from build123d import *

# Parameters (mm, degrees)
ESQUISSE1_R                  = 23
ESQUISSE1_R_2                = 10
BOSS_EXTRU_1_DEPTH           = 8
ENL_V_MAT_EXTRU_1_DEPTH      = 3
ENL_V_MAT_EXTRU_1_DEPTH_BACK = 1
ESQUISSE4_R                  = 4
ENL_V_MAT_EXTRU_2_DEPTH      = 9
R_P_TITION_CIRCULAIRE1_COUNT = 4


with BuildPart() as part:
    # Esquisse1 → Boss.-Extru.1 (new body)
    with BuildSketch(Plane(origin=(0, 0, 0), x_dir=(1, 0, 0), z_dir=(0, 1, 0))):
        with Locations(Location((0, 0, 0), (0, 0, 270))):  # turned: the seam where the file's is
            Circle(ESQUISSE1_R)
        with Locations(Location((0, 0, 0), (0, 0, 270))):  # turned: the seam where the file's is
            Circle(ESQUISSE1_R_2, mode=Mode.SUBTRACT)
    extrude(amount=BOSS_EXTRU_1_DEPTH)

    # Esquisse2 → Enlèv. mat.-Extru.1 (cut, two sides)
    with BuildSketch(Plane.XY.offset(10)) as enl_v_mat_extru_1_sk:
        with BuildLine():
            Line((-3, 0), (-3, 12))
            ThreePointArc((-3, 12), (0, 15), (3, 12))
            Line((3, 12), (3, 0))
            ThreePointArc((3, 0), (0, -3), (-3, 0))
        make_face()
    extrude(amount=ENL_V_MAT_EXTRU_1_DEPTH, mode=Mode.SUBTRACT)
    extrude(enl_v_mat_extru_1_sk.sketch, amount=-ENL_V_MAT_EXTRU_1_DEPTH_BACK, mode=Mode.SUBTRACT)

    # Esquisse4 → Enlèv. mat.-Extru.2 (cut, through all)
    with BuildSketch(Plane.XZ):
        with Locations(Location((12.02081528, 12.02081528, 0), (0, 0, 270))):  # turned: the seam where the file's is
            Circle(ESQUISSE4_R)
    enl_v_mat_extru_2 = extrude(amount=-ENL_V_MAT_EXTRU_2_DEPTH, mode=Mode.SUBTRACT)

    # Répétition circulaire1: Enlèv. mat.-Extru.2 ×4 about axis
    r_p_tition_circulaire1_axis = Axis((0, 0, 0), (0, 1, 0))
    for i in range(1, R_P_TITION_CIRCULAIRE1_COUNT):
        add(enl_v_mat_extru_2.rotate(r_p_tition_circulaire1_axis, i * 360 / R_P_TITION_CIRCULAIRE1_COUNT), mode=Mode.SUBTRACT)


solid = part.part
Source: CAD feature listing. Evaluate the final solid. Frame: model axes, mm. A direction names the side the tool comes from. Give positions to 0.01 mm unless a question says otherwise; leave off trailing zeros. Write each loop counter-clockwise with the first axis right and the second up, starting at its lowest first coordinate (ties: lowest second). Pieces come first, ordered by that corner, then holes. Notation, with made-up numbers: M 39,-17 L 83,-17 A25 cw 83,7 Z; hole C 86,74.25 d10. An arc over 180 degrees is marked long. Return JSON: item names as keys, results as strings. Group by question number.
1) Cut plane A-A, the plane x = 0. Output: boundary loops of the cut face in (y, z), then the cut area to 3 significant figures.
2) Cut plane B-B, the plane z = 0. Output: boundary loops of the cut face in (x, y).
3) Cut plane D-D, the plane x = -19. Output: boundary loops of the cut face in (y, z), then the cut area to 3 significant figures.
4) Cut plane C-C, the plane y = 7. Output: boundary loops of the cut face in (x, z).
5) First-contact query: pin 1 Ø1 at (y, z) = (3, 11.5) entering from -X; pin 2 Ø3 at (y, z) = (1.5, 4.5) entering from +X; pin 3 Ø3 at (y, z) = (6.5, 8.5) entering from +X. Flat tips, straight axial feed; report the tip coordinate or a pass-through.
6) Set-up query: faces 1 (the face through (-5, 8, 10)), 2 (the face through (3, 4, 11)). Return all of +Z, -Z, +X, -X, +Y, -Y with unobstructed straight access to the full face (end or side cutting, diameter ignored); none if empty.
7) Ray query, L1, parallel to X at y = 7.75, z = -14; L2, parallel to X at y = 7.25, z = 8.5; L3, parallel to Z at x = -11.5, y = 7. Return the intervals inside material, ascending.
8) Draft query along X for faces 3 (the face through (-12.542, 3.944, 15.987)), 4 (the face through (-5, 0, 10)), 5 (the face through (19.394, 3.944, 12.365)). Return one class per face: released by +X, released by -X, zero draft, split by the parting line, or undercut.
Data:
{
 "1": {"outline": "M 0,-23 L 8,-23 L 8,-10 L 0,-10 Z; M 0,13 L 8,13 L 8,23 L 0,23 Z", "area": "184 mm²"},
 "2": {"outline": "M -23,0 L -10,0 L -10,8 L -23,8 Z; M 10,0 L 23,0 L 23,8 L 10,8 Z"},
 "3": {"outline": "M 0,-12.96 L 8,-12.96 L 8,12.96 L 0,12.96 Z", "area": "207 mm²"},
 "4": {"outline": "C 0,0 d46; hole C -12.02,-12.02 d8; hole C -12.02,12.02 d8; hole M -3,9.54 A10 ccw long 3,9.54 L 3,13 L -3,13 Z; hole C 12.02,-12.02 d8; hole C 12.02,12.02 d8"},
 "5": {"pin 1": "stops at x = -20.2", "pin 2": "stops at x = 22.8", "pin 3": "stops at x = 21.91"},
 "6": {"face 1": "+Z, -Z, +X, -X, +Y", "face 2": "+Y, -Y"},
 "7": {"L1": "x = -18.25 to -15.5, -8.54 to 8.54, 15.5 to 18.25", "L2": "x = -21.37 to -13.92, -10.12 to -5.27, 5.27 to 10.12, 13.92 to 21.37", "L3": "z = -19.92 to -15.99, -8.05 to 8.05, 15.99 to 19.92"},
 "8": {"face 3": "undercut", "face 4": "zero draft", "face 5": "split by the parting line"}
}
